```python
from build123d import *

# Parameters (mm, degrees)
BOSS_EXTRUDE1_DEPTH = 15
SKETCH3_R           = 2.45
CUT_EXTRUDE1_DEPTH  = 31.822070015
CUT_EXTRUDE2_DEPTH  = 31.822070015


with BuildPart() as part:
    # Sketch2 → Boss-Extrude1 (new body)
    with BuildSketch(Plane.XY):
        with BuildLine():
            Line((-5, 10), (-15, 10))
            ThreePointArc((-15, 10), (-22.071067812, -7.071067812), (-5, 0))
            Line((-5, 0), (5, 0))
            ThreePointArc((5, 0), (22.071067812, -7.071067812), (15, 10))
            Line((15, 10), (5, 10))
            Line((5, 10), (-5, 10))
        make_face()
    extrude(amount=BOSS_EXTRUDE1_DEPTH)

    # Sketch3 → Cut-Extrude1 (cut, through all)
    with BuildSketch(Plane.XY.offset(15)):
        with Locations((-15, 0)):
            Circle(SKETCH3_R)
        with Locations((15, 0)):
            Circle(SKETCH3_R)
    extrude(amount=-CUT_EXTRUDE1_DEPTH, mode=Mode.SUBTRACT)

    # Sketch4 → Cut-Extrude2 (cut, through all)
    with BuildSketch(Plane.XY.offset(15)):
        Polygon((-14.133974596, -0.5), (-15.866025404, 0.5), (-20.866025404, -8.160254038), (-19.133974596, -9.160254038), align=None)
        Polygon((14.133974596, -0.5), (15.866025404, 0.5), (20.866025404, -8.160254038), (19.133974596, -9.160254038), align=None)
    extrude(amount=-CUT_EXTRUDE2_DEPTH, mode=Mode.SUBTRACT)


solid = part.part
```
CAD build for the part. Positions are in the model's coordinates, mm. A direction names the side the tool comes from. Round coordinates to 2 decimals unless told otherwise and drop trailing zeros. Loops run counter-clockwise (first coordinate to the right, second up) from the corner with the lowest first, then second, coordinate; pieces in that order, holes last. Notation, with made-up numbers: M 41.25,36 L 97.25,36 A22 cw 97.25,42 Z; hole C 43.5,16.5 d8. An arc over 180 degrees is marked long. Return JSON: item names as keys, results as strings. Group by question number.
(1) Tool access for faces 5 (the flat face through (-18.886, -4.73, 7.605)), 6 (the flat face through (0, 0, 7)), 7 (the cylindrical face through (24.57, 2.9, 7.4)): list every direction of +Z, -Z, +X, -X, +Y, -Y with a clear straight run to the whole face (end or side of a thin tool).
(2) Saw through at D-D, the plane x = -2. List the corners of the cut face in (y, z).
(3) Mould opens along Y. For faces 1 (the cylindrical face through (-24.46, 3.24, 7.4)), 2 (the cylindrical face through (-13.695, 2.074, 7.605)), 3 (the flat face through (-17.208, -5.824, 7.605)), 4 (the cylindrical face through (9, -8, 7)) say: +Y half, -Y half, draft (parallel to the pull), parting line (faces both ways), or undercut.
(4) Drop flat-ended pins along their axis: P1, Ø3, axis at x = -15, y = 0, coming from the -Z side; P2, Ø1, axis at x = 14, z = 2, coming from the -Y side; P3, Ø3, axis at x = -1, z = 7, coming from the -Y side; P4, Ø2, axis at y = -3.5, z = 6, coming from the -X side. Give the stop position or say it passes through.
(5) Saw through at C-C, the plane z = 11.5. List the corners of the cut face in (x, y).
(6) Saw through at A-A, the plane x = -16. List the corners of the cut face in (y, z), and give its area (3 significant figures).
(7) Saw through at B-B, the plane y = -0.75. List the corners of the cut face in (x, z).
(8) Wall check: probe 1 along Y at (x, z) = (-15, 7); probe 2 along X at (y, z) = (-1.5, 6); probe 3 along X at (y, z) = (-2.75, 3.5). Give the ranges that are in metal, low to high. Write a range as [from, to].
Answer list:
{
 "1": {"face 5": "+Z, -Z", "face 6": "+Z, -Z, -Y", "face 7": "+Z, -Z, +X"},
 "2": {"outline": "M 0,0 L 10,0 L 10,15 L 0,15 Z"},
 "3": {"face 1": "parting line", "face 2": "undercut", "face 3": "undercut", "face 4": "-Y half"},
 "4": {"P1": "through", "P2": "y = -9.99", "P3": "y = 0", "P4": "x = -24.68"},
 "5": {"outline": "M -20.84,-8.12 L -16.98,-1.44 A2.45 cw long -15.25,-2.44 L -19.11,-9.12 A10 ccw -5,0 L 5,0 A10 ccw 19.11,-9.12 L 15.25,-2.44 A2.45 cw long 16.98,-1.44 L 20.84,-8.12 A10 ccw 15,10 L -15,10 A10 ccw Z"},
 "6": {"outline": "M -9.95,0 L -3.73,0 L -3.73,15 L -9.95,15 Z; M 2.24,0 L 9.95,0 L 9.95,15 L 2.24,15 Z", "area": "209 mm2"},
 "7": {"outline": "M -24.97,0 L -17.33,0 L -17.33,15 L -24.97,15 Z; M -12.67,0 L -5.03,0 L -5.03,15 L -12.67,15 Z; M 5.03,0 L 12.67,0 L 12.67,15 L 5.03,15 Z; M 17.33,0 L 24.97,0 L 24.97,15 L 17.33,15 Z"},
 "8": {"probe 1": "[-10, -2.45], [2.45, 10]", "probe 2": "[-24.89, -17.02], [-13.06, -5.11], [5.11, 13.06], [17.02, 24.89]", "probe 3": "[-24.61, -17.74], [-15.43, -5.39], [5.39, 15.43], [17.74, 24.61]"}
}
